Work out the finished part from the listing and answer in its coordinate system (mm). Coordinates: 2 decimals unless noted, no trailing zeros. Order: outer loops, then holes, each group sorted by start corner. A loop starts at its lowest first (then second) coordinate and runs counter-clockwise, first axis right, second up. Notation, with made-up numbers: M 54,-37.75 L 88,-37.75 A11 ccw 88,-30.75 Z; hole C 44.25,34 d2. An arc over 180 degrees is marked long. Answer in a Markdown table with one row per item. Add a question column.
Item 1: The part is cut by section C-C (y = -6.5). Write down the section's boundary in (x, z), then the cut area to 3 significant figures.
Item 2: Consider line 1 (Z direction, x = 0, y = -3); line 2 (X direction, y = 0, z = -0.5). Determine where each line is inside the solid, lowest interval first. Write a range as from..to.
Item 3: The part is cut by section A-A (z = -1). Write down the section's boundary in (x, y).
Item 4: The part is cut by section B-B (x = 0). Write down the section's boundary in (y, z).
Item 5: The mould has two halves that part along Z. Classify faces 1 (the face through (4.23, -0.11, -4.2)), 2 (the face through (0, 0, 4.8)), 3 (the face through (1.717, -0.105, -0.541)), 4 (the face through (2, -7.5, 0)): released by +Z, released by -Z, zero draft, split by the parting line, or undercut.
Item 6: A flat-ended cylindrical pin translates along its axis: pin 1 Ø1.5 at (y, z) = (3.5, -4) entering from +X. Find the tip coordinate at first contact, or state that the pin passes through.
Item 7: The part is cut by section D-D (z = 4.25). Write down the section's boundary in (x, y).
from build123d import *

# Parameters (mm, degrees)
SKETCH1_W           = 9.6
SKETCH1_H           = 9.6
SKETCH1_R           = 1.8
BOSS_EXTRUDE1_DEPTH = 7.5
FILLET1_R           = 2


with BuildPart() as part:
    # Sketch1 → Boss-Extrude1 (new body, symmetric)
    with BuildSketch(Plane(origin=(0, 0, 0), x_dir=(1, 0, 0), z_dir=(0, 1, 0))):
        Rectangle(SKETCH1_W, SKETCH1_H)
        Circle(SKETCH1_R, mode=Mode.SUBTRACT)
    extrude(amount=BOSS_EXTRUDE1_DEPTH, both=True)

    # Fillet1
    fillet1_edges = [part.edges().sort_by_distance(p)[0] for p in [
        (-4.8, 0, -4.8),
        (4.8, 0, -4.8),
        (4.8, 0, 4.8),
        (-4.8, 0, 4.8),
    ]]
    fillet(fillet1_edges, radius=FILLET1_R)


solid = part.part
Reply:
| question | item | result |
|---|---|---|
| 1 | outline | M -4.8,-2.8 A2 ccw -2.8,-4.8 L 2.8,-4.8 A2 ccw 4.8,-2.8 L 4.8,2.8 A2 ccw 2.8,4.8 L -2.8,4.8 A2 ccw -4.8,2.8 Z; hole C 0,0 d3.6 |
| 1 | area | 78.5 mm2 |
| 2 | line 1 | z = -4.8..-1.8, 1.8..4.8 |
| 2 | line 2 | x = -4.8..-1.73, 1.73..4.8 |
| 3 | outline | M -4.8,-7.5 L -1.5,-7.5 L -1.5,7.5 L -4.8,7.5 Z; M 1.5,-7.5 L 4.8,-7.5 L 4.8,7.5 L 1.5,7.5 Z |
| 4 | outline | M -7.5,-4.8 L 7.5,-4.8 L 7.5,-1.8 L -7.5,-1.8 Z; M -7.5,1.8 L 7.5,1.8 L 7.5,4.8 L -7.5,4.8 Z |
| 5 | face 1 | released by -Z |
| 5 | face 2 | released by +Z |
| 5 | face 3 | undercut |
| 5 | face 4 | zero draft |
| 6 | pin 1 | stops at x = 4.75 |
| 7 | outline | M -4.18,-7.5 L 4.18,-7.5 L 4.18,7.5 L -4.18,7.5 Z |
